Check sheet for the modelled part. Datum: model origin and axes. Units: mm. Face numbers are marked on the shaded views. Give positions to 0.01 mm unless a question says otherwise; leave off trailing zeros. Order: outer loops, then holes, each group sorted by start corner. A loop starts at its lowest first (then second) coordinate and runs counter-clockwise, first axis right, second up.
Autodesk Inventor part; units mm, degrees
ref_plane "YZ Plane" through (0, 0, 0) normal (1, 0, 0) x (0, 1, 0)
ref_plane "XZ Plane" through (0, 0, 0) normal (0, 1, 0) x (-1, 0, 0)
ref_plane "XY Plane" through (0, 0, 0) normal (0, 0, 1) x (1, 0, 0)
sketch "Skizze1" plane through (0, 0, 0) normal (1, 0, 0) x (0, 1, 0)
  line L0 (300, 30) -> (250, 30)
  line L1 (250, 30) -> (250, 0)
  line L2 (250, 0) -> (300, 0)
  line L3 (300, 0) -> (300, 30)
  line L4 (-250, 30) -> (-300, 30)
  line L5 (-300, 30) -> (-300, 0)
  line L6 (-300, 0) -> (-250, 0)
  line L7 (-250, 0) -> (-250, 30)
  line L8 (300, 0) -> (-300, 0)
  line L9 (-300, 0) -> (-300, -10)
  line L10 (-300, -10) -> (300, -10)
  line L11 (300, -10) -> (300, 0)
  point P0 (0, 0)
  point P1 (0, 0)
  point P2 (250, 0)
  point P3 (-250, 0)
  dimension "d0" = 50
  dimension "d1" = 30
  dimension "d2" = 600
  dimension "d3" = 10
extrude "Extrusion1" add sketch "Skizze1" along normal mid plane 700
properties part number "Drawer" material "Holz (Birke)"
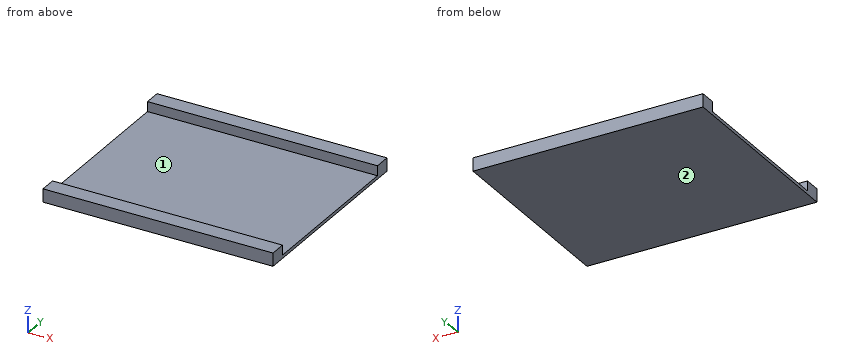
(1) Release check for a two-part mould opening along Y. For the marked faces 1 and 2 record: released by +Y, released by -Y, zero draft, split by the parting line, or undercut.
(2) Sectioned sample at B-B (x = -191). Enter the section's corners in (y, z), plus the area to 3 significant figures.
(3) Thickness scan on L1, parallel to Y at x = -104, z = 17; L2, parallel to Z at x = -238.5, y = -192. Record the ranges inside material, lowest first.
(4) Sectioned sample at C-C (y = 58). Enter the section's corners in (x, z).
(5) Sectioned sample at A-A (z = 16). Enter the section's corners in (x, y).
(6) Go/stop test with a flat-tipped pin: P1, Ø10, axis at x = -21.5, y = 166, coming from the +Z side. Record where the tip stops, or that it passes through.
Values follow:
1. face 1: undercut
1. face 2: zero draft
2. outline: (-300, -10) - (300, -10) - (300, 30) - (250, 30) - (250, 0) - (-250, 0) - (-250, 30) - (-300, 30) - close
2. area: 9,000 mm2
3. L1: y = -300 to -250, 250 to 300
3. L2: z = -10 to 0
4. outline: (-350, -10) - (350, -10) - (350, 0) - (-350, 0) - close
5. outline: (-350, -300) - (350, -300) - (350, -250) - (-350, -250) - close; (-350, 250) - (350, 250) - (350, 300) - (-350, 300) - close
6. P1: stops at z = 0
